Here's how the part is built. I have some questions about the finished solid (model axes, mm). A direction names the side the tool comes from. Round coordinates to 2 decimals unless told otherwise and drop trailing zeros. Write each loop counter-clockwise with the first axis right and the second up, starting at its lowest first coordinate (ties: lowest second). Pieces come first, ordered by that corner, then holes. Notation, with made-up numbers: (1, 53) -> (8, 53) arc R12 ccw to (8, 72) -> close; hole circle Ø10 at (2.25, 65). An arc over 180 degrees is marked (long way). Answer as CSV lines item,"result".
from build123d import *

# Parameters (mm, degrees)
F1_DEPTH = 19
F2_W     = 190
F2_H     = 19
F3_DEPTH = 19
F4_W     = 190
F4_H     = 19
F5_DEPTH = 19


with BuildPart() as f1:
    # F0 (on Top) → F1 (new body)
    with BuildSketch(Plane.XY):
        Polygon((0, 150), (0, 0), (980, 0), (980, 150), (790, 390), (190, 390), align=None)
    extrude(amount=F1_DEPTH)

    # F2 (on face) → F3 (cut)
    with BuildSketch(Plane.XY.offset(19)):
        with Locations((95, 9.5)):
            Rectangle(F2_W, F2_H)
    extrude(amount=-F3_DEPTH, mode=Mode.SUBTRACT)

    # F4 (on face) → F5 (cut)
    with BuildSketch(Plane.XY.offset(19)):
        with Locations((885, 9.5)):
            Rectangle(F4_W, F4_H)
    extrude(amount=-F5_DEPTH, mode=Mode.SUBTRACT)


solid = f1.part
Item 1: I need wall thicknesses on L1, parallel to X at y = 275.5, z = 3.75; L2, parallel to X at y = 210, z = 18; L3, parallel to Y at x = 897.5, z = 16. Which ranges of each line are inside material? Lowest first, please.
Results found:
L1,"x = 99.35 to 880.65"
L2,"x = 47.5 to 932.5"
L3,"y = 19 to 254.21"
Item 2: For faces 1 (the flat face through (94, 19, 10)), 2 (the flat face through (790, 9, 10)), 3 (the flat face through (886.33, 268.32, 9.37)), which set-ups out of +Z, -Z, +X, -X, +Y, -Y let a thin tool reach every point of the face, with its end or its side?
Results found:
face 1,"+Z, -Z, -X, -Y"
face 2,"+Z, -Z, +X, -Y"
face 3,"+Z, -Z, +X, +Y"
Item 3: Suppose I cut it at A-A, the plane z = 15.5. List the corners of the cut face in (x, y) for me, then the cut area to 3 significant figures.
Results found:
outline,"(0, 19) -> (190, 19) -> (190, 0) -> (790, 0) -> (790, 19) -> (980, 19) -> (980, 150) -> (790, 390) -> (190, 390) -> (0, 150) -> close"
area,"329,000 mm²"
Item 4: Will these pins go through, and if not, where does the flat tip stop? pin 1 (4 mm diameter, centred on y = 274.5, z = 9.5, fed in from -X); pin 2 (9.5 mm diameter, centred on y = 9, z = 11.5, fed in from -X); pin 3 (5.5 mm diameter, centred on x = 62.5, z = 8, fed in from -Y).
Results found:
pin 1,"stops at x = 96.98"
pin 2,"stops at x = 190"
pin 3,"stops at y = 19"
Item 5: Suppose I cut it at C-C, the plane x = 95. List the corners of the cut face in (y, z) for me, then the cut area to 3 significant figures.
Results found:
outline,"(19, 0) -> (270, 0) -> (270, 19) -> (19, 19) -> close"
area,"4,770 mm²"
Item 6: Suppose I cut it at B-B, the plane y = 211. List the corners of the cut face in (x, z) for me, then the cut area to 3 significant figures.
Results found:
outline,"(48.29, 0) -> (931.71, 0) -> (931.71, 19) -> (48.29, 19) -> close"
area,"16,800 mm²"
